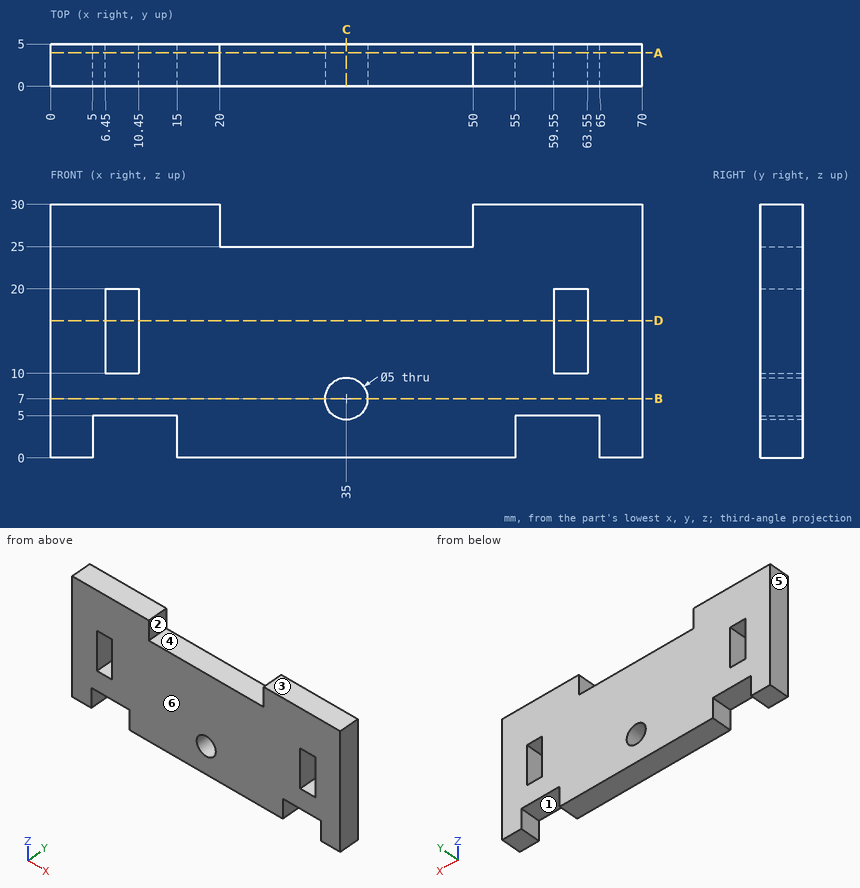
Check sheet for the drawn part. Datum: minimum x, y, z corner. Units: mm. A direction names the side the tool comes from. Round coordinates to 2 decimals unless told otherwise and drop trailing zeros. Order: outer loops, then holes, each group sorted by start corner. A loop starts at its lowest first (then second) coordinate and runs counter-clockwise, first axis right, second up. Notation, with made-up numbers: (27.25, 30.25) - (44.25, 30.25) arc R30 cw to (44.25, 60.25) - close; hole circle Ø11 at (17, -3). An arc over 180 degrees is marked (long way). Use a Markdown table: item, result. Add a question column.
(1) Material ranges on line 1 along X through (y, z) = (4.4, 10.25); line 2 along X through (y, z) = (3.9, 27); line 3 along X through (y, z) = (1.2, 7), recorded low to high. Write a range as [from, to].
(2) Depth check by flat-ended pin: pin 1 (4.5 mm diameter, centred on x = 35, z = 7, fed in from -Y); pin 2 (2 mm diameter, centred on x = 61, y = 2.5, fed in from -Z). Enter the tip coordinate at first touch or a pass-through.
(3) Sectioned sample at A-A, the plane y = 3.95. Enter the section's corners in (x, z), and give its area (3 significant figures).
(4) Sectioned sample at C-C, the plane x = 35. Enter the section's corners in (y, z), and give its area (3 significant figures).
(5) Sectioned sample at D-D, the plane z = 16.25. Enter the section's corners in (x, y), and give its area (3 significant figures).
(6) Sectioned sample at B-B, the plane z = 7. Enter the section's corners in (x, y).
(7) Tool access check on the marked faces 1, 2 and 3. Record the directions out of +Z, -Z, +X, -X, +Y, -Y that give a thin tool (end or side, any length) a straight path to the whole face; none if there is none.
(8) Release check for a two-part mould opening along X. For the marked faces 4, 5 and 6 record: pulls with the +X half, pulls with the -X half, needs draft (parallel to the pull), parting line crosses it, or undercut.
Answers below:
| question | item | result |
|---|---|---|
| 1 | line 1 | [0, 6.45], [10.45, 59.55], [63.55, 70] |
| 1 | line 2 | [0, 20], [50, 70] |
| 1 | line 3 | [0, 32.5], [37.5, 70] |
| 2 | pin 1 | through |
| 2 | pin 2 | z = 5 |
| 3 | outline | (0, 0) - (5, 0) - (5, 5) - (15, 5) - (15, 0) - (55, 0) - (55, 5) - (65, 5) - (65, 0) - (70, 0) - (70, 30) - (50, 30) - (50, 25) - (20, 25) - (20, 30) - (0, 30) - close; hole (6.45, 10) - (10.45, 10) - (10.45, 20) - (6.45, 20) - close; hole circle Ø5 at (35, 7); hole (59.55, 10) - (63.55, 10) - (63.55, 20) - (59.55, 20) - close |
| 3 | area | 1,750 mm² |
| 4 | outline | (0, 0) - (5, 0) - (5, 4.5) - (0, 4.5) - close; (0, 9.5) - (5, 9.5) - (5, 25) - (0, 25) - close |
| 4 | area | 100 mm² |
| 5 | outline | (0, 0) - (6.45, 0) - (6.45, 5) - (0, 5) - close; (10.45, 0) - (59.55, 0) - (59.55, 5) - (10.45, 5) - close; (63.55, 0) - (70, 0) - (70, 5) - (63.55, 5) - close |
| 5 | area | 310 mm² |
| 6 | outline | (0, 0) - (32.5, 0) - (32.5, 5) - (0, 5) - close; (37.5, 0) - (70, 0) - (70, 5) - (37.5, 5) - close |
| 7 | face 1 | -Z, +Y, -Y |
| 7 | face 2 | +Z, +Y, -Y |
| 7 | face 3 | +Z, +X, -X, +Y, -Y |
| 8 | face 4 | undercut |
| 8 | face 5 | pulls with the -X half |
| 8 | face 6 | needs draft |
